Input: part model. Units: mm. Frame: model coordinates. Round coordinates to 2 decimals unless told otherwise and drop trailing zeros. Write each loop counter-clockwise with the first axis right and the second up, starting at its lowest first coordinate (ties: lowest second). Pieces come first, ordered by that corner, then holes. Notation, with made-up numbers: M 82.5,-10 L 88.5,-10 A12 ccw 88.5,-6 Z; hole C 3.25,79.25 d1. An arc over 180 degrees is marked long. Use one line per item in the form item = value. Start each with the question number.
```python
from build123d import *

# Parameters (mm, degrees)
SKETCH1_W           = 140
SKETCH1_H           = 300
SKETCH1_R           = 2.125
BOSS_EXTRUDE1_DEPTH = 6.35
SKETCH2_R           = 12
SKETCH2_R_2         = 2.125
CUT_EXTRUDE1_DEPTH  = 166.651207361


with BuildPart() as part:
    # Sketch1 → Boss-Extrude1 (new body)
    with BuildSketch(Plane.XY):
        Rectangle(SKETCH1_W, SKETCH1_H)
        with Locations((-62, 138.825)):
            Circle(SKETCH1_R, mode=Mode.SUBTRACT)
        with Locations(Location((-38, 138.825, 0), (0, 0, 180))):
            Circle(SKETCH1_R, mode=Mode.SUBTRACT)
        with Locations((-38, 114.825)):
            Circle(SKETCH1_R, mode=Mode.SUBTRACT)
        with Locations(Location((-62, 114.825, 0), (0, 0, 180))):
            Circle(SKETCH1_R, mode=Mode.SUBTRACT)
        with Locations(Location((38, 114.825, 0), (0, 0, 180))):
            Circle(SKETCH1_R, mode=Mode.SUBTRACT)
        with Locations((62, 114.825)):
            Circle(SKETCH1_R, mode=Mode.SUBTRACT)
        with Locations((38, 138.825)):
            Circle(SKETCH1_R, mode=Mode.SUBTRACT)
        with Locations(Location((62, 138.825, 0), (0, 0, 180))):
            Circle(SKETCH1_R, mode=Mode.SUBTRACT)
        with Locations((62, -46.825)):
            Circle(SKETCH1_R, mode=Mode.SUBTRACT)
        with Locations(Location((38, -46.825, 0), (0, 0, 180))):
            Circle(SKETCH1_R, mode=Mode.SUBTRACT)
        with Locations(Location((62, -22.825, 0), (0, 0, 180))):
            Circle(SKETCH1_R, mode=Mode.SUBTRACT)
        with Locations((38, -22.825)):
            Circle(SKETCH1_R, mode=Mode.SUBTRACT)
        with Locations((-62, -22.825)):
            Circle(SKETCH1_R, mode=Mode.SUBTRACT)
        with Locations(Location((-38, -22.825, 0), (0, 0, 180))):
            Circle(SKETCH1_R, mode=Mode.SUBTRACT)
        with Locations((-38, -46.825)):
            Circle(SKETCH1_R, mode=Mode.SUBTRACT)
        with Locations(Location((-62, -46.825, 0), (0, 0, 180))):
            Circle(SKETCH1_R, mode=Mode.SUBTRACT)
        with Locations((-62, -111.175)):
            Circle(SKETCH1_R, mode=Mode.SUBTRACT)
        with Locations(Location((-38, -111.175, 0), (0, 0, 180))):
            Circle(SKETCH1_R, mode=Mode.SUBTRACT)
        with Locations((-38, -135.175)):
            Circle(SKETCH1_R, mode=Mode.SUBTRACT)
        with Locations(Location((-62, -135.175, 0), (0, 0, 180))):
            Circle(SKETCH1_R, mode=Mode.SUBTRACT)
        with Locations(Location((38, -135.175, 0), (0, 0, 180))):
            Circle(SKETCH1_R, mode=Mode.SUBTRACT)
        with Locations((62, -135.175)):
            Circle(SKETCH1_R, mode=Mode.SUBTRACT)
        with Locations((38, -111.175)):
            Circle(SKETCH1_R, mode=Mode.SUBTRACT)
        with Locations(Location((62, -111.175, 0), (0, 0, 180))):
            Circle(SKETCH1_R, mode=Mode.SUBTRACT)
    extrude(amount=BOSS_EXTRUDE1_DEPTH)

    # Sketch2 → Cut-Extrude1 (cut, through all)
    with BuildSketch(Plane.XY.offset(6.35)):
        with Locations((0, -33.35)):
            Circle(SKETCH2_R)
        with Locations((-1.565325907, -13.411350226)):
            Circle(SKETCH2_R_2)
        with Locations((18.050040175, -41.963712886)):
            Circle(SKETCH2_R_2)
        with Locations((-16.484714268, -44.674936888)):
            Circle(SKETCH2_R_2)
    extrude(amount=-CUT_EXTRUDE1_DEPTH, mode=Mode.SUBTRACT)


solid = part.part
```
Item 1: Cut plane B-B (z = 4.25). Give the number of separate pieces and of enclosed holes in the cut face, plus the area to 3 significant figures.
Item 2: Cut plane A-A (y = -33.35). Output: boundary loops of the cut face in (x, z), plus the area to 3 significant figures.
Item 3: Ray query, line 1 (Y direction, x = -10, z = 3); line 2 (Y direction, x = -7, z = 1.25). Return the intervals inside material, ascending. Write a range as from..to.
Item 4: First-contact query: pin 1 (3.5 mm diameter, centred on x = -38, y = 138.825, fed in from +Z). Flat tip, straight axial feed; report the tip coordinate or a pass-through.
Final values:
q1.separate_pieces = 1
q1.enclosed_holes = 28
q1.area = 41,200 mm^2
q2.outline = M -70,0 L -12,0 L -12,6.35 L -70,6.35 Z; M 12,0 L 70,0 L 70,6.35 L 12,6.35 Z
q2.area = 737 mm^2
q3.line_1 = -150..-39.98, -26.72..150
q3.line_2 = -150..-43.1, -23.6..150
q4.pin_1 = through
